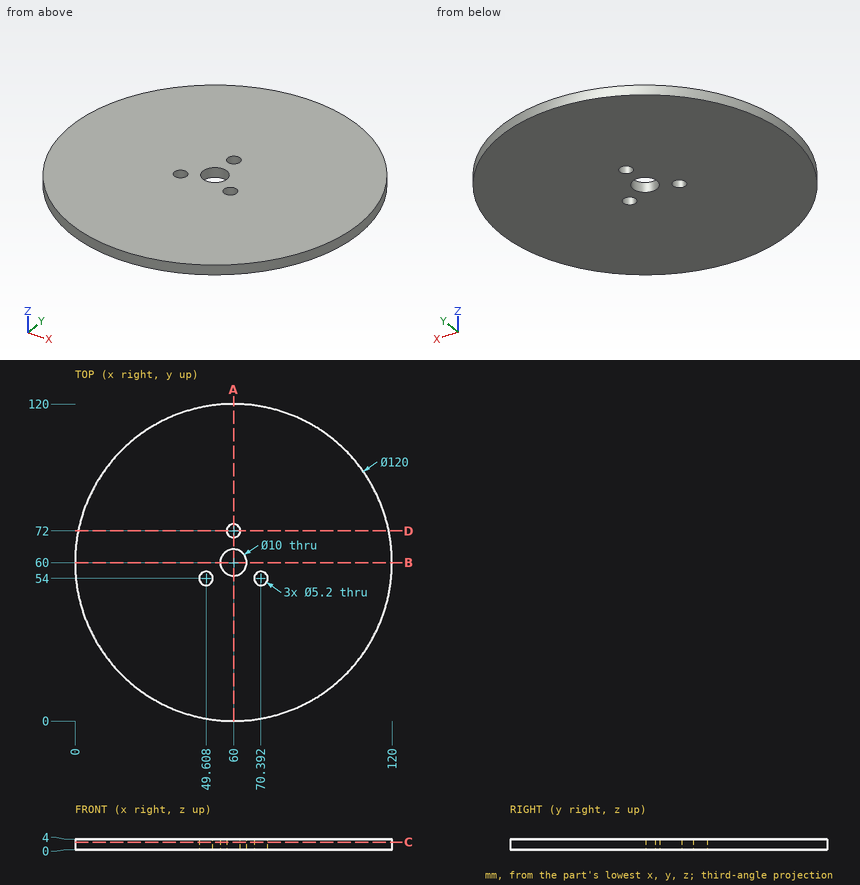
Geometry: see drawing. Coordinates: mm, zero at the bounding-box minimum. Give positions to 0.01 mm unless a question says otherwise; leave off trailing zeros. Order: outer loops, then holes, each group sorted by start corner. A loop starts at its lowest first (then second) coordinate and runs counter-clockwise, first axis right, second up. Notation, with made-up numbers: (17.25, 62) - (63.25, 62) arc R19 ccw to (63.25, 78) - close; hole circle Ø1 at (46, 11). An arc over 180 degrees is marked (long way). Use a Markdown table: item, result.
(1) Section query B-B (y = 60). Output: boundary loops of the cut face in (x, z).
Computed values:
| item | result |
|---|---|
| outline | (0, 0) - (55, 0) - (55, 4) - (0, 4) - close; (65, 0) - (120, 0) - (120, 4) - (65, 4) - close |
(2) Section query A-A (x = 60). Output: boundary loops of the cut face in (y, z), then the cut area to 3 significant figures.
Computed values:
| item | result |
|---|---|
| outline | (0, 0) - (55, 0) - (55, 4) - (0, 4) - close; (65, 0) - (69.4, 0) - (69.4, 4) - (65, 4) - close; (74.6, 0) - (120, 0) - (120, 4) - (74.6, 4) - close |
| area | 419 mm2 |
(3) Section query C-C (z = 2.85). Output: boundary loops of the cut face in (x, y), then the cut area to 3 significant figures.
Computed values:
| item | result |
|---|---|
| outline | circle Ø120 at (60, 60); hole circle Ø5.2 at (49.61, 54); hole circle Ø10 at (60, 60); hole circle Ø5.2 at (60, 72); hole circle Ø5.2 at (70.39, 54) |
| area | 11,200 mm2 |
(4) Section query D-D (y = 72). Output: boundary loops of the cut face in (x, z).
Computed values:
| item | result |
|---|---|
| outline | (1.21, 0) - (57.4, 0) - (57.4, 4) - (1.21, 4) - close; (62.6, 0) - (118.79, 0) - (118.79, 4) - (62.6, 4) - close |
(5) Line query: line 1 (Y direction, x = 60, z = 0.8); line 2 (X direction, y = 53.5, z = 3.8); line 3 (X direction, y = 102.5, z = 1). Output: solid intervals per line, ascending. Write a range as from..to.
Computed values:
| item | result |
|---|---|
| line 1 | y = 0..55, 65..69.4, 74.6..120 |
| line 2 | x = 0.35..47.06, 52.16..67.84, 72.94..119.65 |
| line 3 | x = 17.65..102.35 |
